```python
from build123d import *

# Parameters (mm, degrees)
SKETCH1_W           = 26
SKETCH1_H           = 10
BOSS_EXTRUDE1_DEPTH = 13
SKETCH2_R           = 7.6
CUT_EXTRUDE1_DEPTH  = 20.052558883
SKETCH3_R           = 1.65
CUT_EXTRUDE2_DEPTH  = 10
FILLET2_R           = 4


with BuildPart() as part:
    # Sketch1 → Boss-Extrude1 (new body)
    with BuildSketch(Plane.XY):
        Rectangle(SKETCH1_W, SKETCH1_H)
    extrude(amount=BOSS_EXTRUDE1_DEPTH)

    # Sketch2 → Cut-Extrude1 (cut, through all)
    with BuildSketch(Plane.XY.offset(13)):
        with Locations((0, 6)):
            Circle(SKETCH2_R)
    extrude(amount=-CUT_EXTRUDE1_DEPTH, mode=Mode.SUBTRACT)

    # Sketch3 → Cut-Extrude2 (cut)
    with BuildSketch(Plane(origin=(0, 5, 0), x_dir=(1, 0, 0), z_dir=(0, 1, 0))):
        with Locations(Location((-10.26696164, -6.5, 0), (0, 0, 270))):
            Circle(SKETCH3_R)
        with Locations(Location((10.26696164, -6.5, 0), (0, 0, 270))):
            Circle(SKETCH3_R)
    extrude(amount=-CUT_EXTRUDE2_DEPTH, mode=Mode.SUBTRACT)

    # Fillet2
    fillet2_edges = [part.edges().sort_by_distance(p)[0] for p in [
        (-13, 0, 13),
        (13, 0, 13),
        (-13, 0, 0),
        (13, 0, 0),
    ]]
    fillet(fillet2_edges, radius=FILLET2_R)


solid = part.part
```
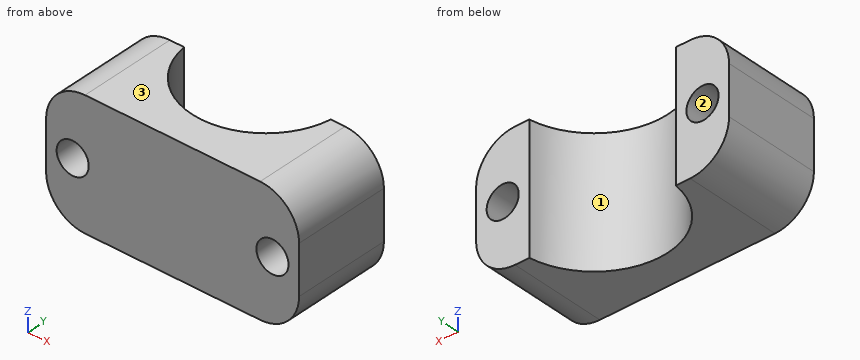
Check sheet for the modelled part. Datum: model origin and axes. Units: mm. Face numbers are marked on the shaded views. Give positions to 0.01 mm unless a question says otherwise; leave off trailing zeros. Loops run counter-clockwise (first coordinate to the right, second up) from the corner with the lowest first, then second, coordinate; pieces in that order, holes last. Notation, with made-up numbers: M -33.5,3 L -2.5,3 A24 ccw -2.5,39 Z; hole C -36,55 d6. An arc over 180 degrees is marked long. Answer in a Markdown table with one row per item.
1) Mould release check, pull along Z, two halves, no side actions. Record for the marked faces 1, 2 and 3: released by +Z, released by -Z, zero draft, split by the parting line, or undercut.
Solutions:
| item | result |
|---|---|
| face 1 | zero draft |
| face 2 | undercut |
| face 3 | released by +Z |
2) Cross-section at C-C (x = 11.25). Enter the section's corners in (y, z), plus the area to 3 significant figures.
Solutions:
| item | result |
|---|---|
| outline | M -5,0.69 L 5,0.69 L 5,5.17 L -5,5.17 Z; M -5,7.83 L 5,7.83 L 5,12.31 L -5,12.31 Z |
| area | 89.6 mm^2 |
3) Cross-section at A-A (z = 6.5). Enter the section's corners in (x, y), plus the area to 3 significant figures.
Solutions:
| item | result |
|---|---|
| outline | M -13,-5 L -11.92,-5 L -11.92,5 L -13,5 Z; M -8.62,-5 L 8.62,-5 L 8.62,5 L 7.53,5 A7.6 cw -7.53,5 L -8.62,5 Z; M 11.92,-5 L 13,-5 L 13,5 L 11.92,5 Z |
| area | 118 mm^2 |
4) Cross-section at B-B (y = 2.5). Enter the section's corners in (x, z), plus the area to 3 significant figures.
Solutions:
| item | result |
|---|---|
| outline | M -13,4 A4 ccw -9,0 L -6.75,0 L -6.75,13 L -9,13 A4 ccw -13,9 Z; M 6.75,0 L 9,0 A4 ccw 13,4 L 13,9 A4 ccw 9,13 L 6.75,13 Z; hole C -10.27,6.5 d3.3; hole C 10.27,6.5 d3.3 |
| area | 132 mm^2 |
5) Thickness scan on line 1 (X direction, y = -2, z = 6.5); line 2 (X direction, y = 0.75, z = 6.5); line 3 (X direction, y = -0.25, z = 6.5). Record the ranges inside material, lowest first.
Solutions:
| item | result |
|---|---|
| line 1 | x = -13 to -11.92, -8.62 to 8.62, 11.92 to 13 |
| line 2 | x = -13 to -11.92, -8.62 to -5.5, 5.5 to 8.62, 11.92 to 13 |
| line 3 | x = -13 to -11.92, -8.62 to -4.32, 4.32 to 8.62, 11.92 to 13 |
6) Cross-section at D-D (y = 1). Enter the section's corners in (x, z).
Solutions:
| item | result |
|---|---|
| outline | M -13,4 A4 ccw -9,0 L -5.72,0 L -5.72,13 L -9,13 A4 ccw -13,9 Z; M 5.72,0 L 9,0 A4 ccw 13,4 L 13,9 A4 ccw 9,13 L 5.72,13 Z; hole C -10.27,6.5 d3.3; hole C 10.27,6.5 d3.3 |
